Verification items for the finished model (mm, model axes). Face numbers are marked on the shaded views. A direction names the side the tool comes from. Give positions to 0.01 mm unless a question says otherwise; leave off trailing zeros. Write each loop counter-clockwise with the first axis right and the second up, starting at its lowest first coordinate (ties: lowest second). Pieces come first, ordered by that corner, then holes. Notation, with made-up numbers: (7.5, 33) - (63.5, 33) arc R18 ccw to (63.5, 68) - close; hole circle Ø9 at (-9.5, 59). An arc over 180 degrees is marked (long way). Answer as a JSON object with one key per item and string values. Group by question number.
Item 1: Sectioned sample at C-C, the plane x = 0. Record the boundary of the cut face in (y, z), and give its area (3 significant figures).
Item 2: Sectioned sample at A-A, the plane z = 0. Record the boundary of the cut face in (x, y).
Item 3: Scan lines: line 1 along Y through (x, z) = (3.25, 2.5); line 2 along X through (y, z) = (13, 2.5); line 3 along Z through (x, y) = (-1.5, -3.5). Record each from-to range of solid material in increasing order. Write a range as [from, to].
Item 4: Sectioned sample at D-D, the plane y = -3. Record the boundary of the cut face in (x, z), and give its area (3 significant figures).
Item 5: Sectioned sample at B-B, the plane y = 20.5. Record the boundary of the cut face in (x, z), and give its area (3 significant figures).
Item 6: Go/stop test with flat-tipped pins: pin 1 (4 mm diameter, centred on x = -5, y = 18, fed in from -Z); pin 2 (8 mm diameter, centred on x = -1.5, z = -10, fed in from +Y); pin 3 (7.5 mm diameter, centred on x = 0, y = -4.5, fed in from +Z). Record where each tip stops, or that it passes through.
Item 7: Tool access check on the marked faces 1, 2 and 3. Record the directions out of +Z, -Z, +X, -X, +Y, -Y that give a thin tool (end or side, any length) a straight path to the whole face; none if there is none.
```python
from build123d import *

# Parameters (mm, degrees)
SKETCH1_R                = 13.8
BOSS_EXTRUDE1_DEPTH      = 18
SKETCH3_R                = 2.5
BOSS_EXTRUDE2_DEPTH      = 12.7
BOSS_EXTRUDE3_DEPTH      = 11
BOSS_EXTRUDE3_DEPTH_BACK = 3


with BuildPart() as part:
    # Sketch1 → Boss-Extrude1 (new body)
    with BuildSketch(Plane(origin=(0, 0, 0), x_dir=(1, 0, 0), z_dir=(0, 1, 0))):
        with Locations(Location((0, 0, 0), (0, 0, 270))):
            Circle(SKETCH1_R)
    extrude(amount=BOSS_EXTRUDE1_DEPTH)

    # Sketch2 → Cut-Revolve1 (revolve, cut)
    with BuildSketch(Plane(origin=(0, 0, 0), x_dir=(0, 0, -1), z_dir=(1, 0, 0)), mode=Mode.PRIVATE) as cut_revolve1_sk:
        Polygon((12.032233047, 18), (13.8, 16.232233047), (13.8, 18), align=None)
        Polygon((13.8, 0), (13.8, 1.767766953), (12.032233047, 0), align=None)
    revolve(cut_revolve1_sk.sketch.rotate(Axis((0, 18, 0), (0, -1, 0)), 180), axis=Axis((0, 18, 0), (0, -1, 0)), mode=Mode.SUBTRACT)

    # Sketch3 → Boss-Extrude2 (add)
    with BuildSketch(Plane(origin=(0, 18, 0), x_dir=(1, 0, 0), z_dir=(0, 1, 0))):
        with Locations(Location((0, 0, 0), (0, 0, 270))):
            Circle(SKETCH3_R)
    extrude(amount=BOSS_EXTRUDE2_DEPTH)

    # Sketch4 → Boss-Extrude3 (add, two sides: drawn at the far end of the back side and taken through both)
    with BuildSketch(Plane.XZ.offset(-BOSS_EXTRUDE3_DEPTH_BACK)):
        with BuildLine():
            Line((3.5, 12.75), (-3.5, 12.75))
            Line((-3.5, 12.75), (-3.5, 11.511934333))
            ThreePointArc((-3.5, 11.511934333), (0, 12.032233047), (3.5, 11.511934333))
            Line((3.5, 11.511934333), (3.5, 12.75))
        make_face()
        with BuildLine():
            ThreePointArc((3.5, 11.511934333), (0, 12.032233047), (-3.5, 11.511934333))
            Line((-3.5, 11.511934333), (-3.5, 9.75))
            Line((-3.5, 9.75), (0, 9.75))
            Line((0, 9.75), (3.5, 9.75))
            Line((3.5, 9.75), (3.5, 11.511934333))
        make_face()
    extrude(amount=BOSS_EXTRUDE3_DEPTH + BOSS_EXTRUDE3_DEPTH_BACK)


solid = part.part
```
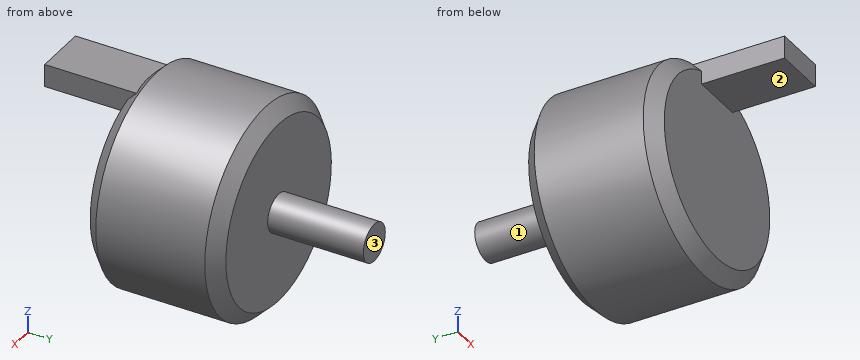
Geometry check:
{
 "1": {"outline": "(-11, 9.75) - (0, 9.75) - (0, -12.03) - (1.77, -13.8) - (16.23, -13.8) - (18, -12.03) - (18, -2.5) - (30.7, -2.5) - (30.7, 2.5) - (18, 2.5) - (18, 12.03) - (16.23, 13.8) - (1.77, 13.8) - (0.72, 12.75) - (-11, 12.75) - close", "area": "587 mm^2"},
 "2": {"outline": "(-13.8, 1.77) - (-12.03, 0) - (12.03, 0) - (13.8, 1.77) - (13.8, 16.23) - (12.03, 18) - (2.5, 18) - (2.5, 30.7) - (-2.5, 30.7) - (-2.5, 18) - (-12.03, 18) - (-13.8, 16.23) - close"},
 "3": {"line 1": "[0, 18]", "line 2": "[-13.57, 13.57]", "line 3": "[9.75, 12.75]"},
 "4": {"outline": "(-3.5, 9.75) - (3.5, 9.75) - (3.5, 12.75) - (-3.5, 12.75) - close", "area": "21.0 mm^2"},
 "5": {"outline": "circle Ø5 at (0, 0)", "area": "19.6 mm^2"},
 "6": {"pin 1": "z = -13.19", "pin 2": "y = 18", "pin 3": "z = 12.75"},
 "7": {"face 1": "+Y", "face 2": "-Z, +X, -X, -Y", "face 3": "+Z, -Z, +X, -X, +Y"}
}
